```python
from build123d import *

# Parameters (mm, degrees)
BOSS_EXTRUDE1_DEPTH = 7.5
CIRPATTERN1_COUNT   = 20


with BuildPart() as part:
    # Sketch1 → Revolve1 (revolve)
    with BuildSketch(Plane(origin=(0, 0, 0), x_dir=(0, 0, -1), z_dir=(1, 0, 0)), mode=Mode.PRIVATE) as revolve1_sk:
        Polygon((-3.75, 7.5), (-3.75, 5.5), (3.75, 5.5), (3.75, 7.5), (4.25, 9), (5.4, 9), (5.4, 5.075), (5.8, 5.075), (5.8, 2.5), (-5.8, 2.5), (-5.8, 5.075), (-5.4, 5.075), (-5.4, 9), (-4.25, 9), align=None)
    revolve(revolve1_sk.sketch.rotate(Axis((0, 0, 0), (0, 0, -1)), 90), axis=Axis((0, 0, 0), (0, 0, -1)))

    # Sketch2 → Boss-Extrude1 (add)
    with BuildSketch(Plane.XY.offset(-3.75)):
        with BuildLine():
            ThreePointArc((0.499483204, 5.477272727), (0, 6), (-0.499483204, 5.477272727))
            ThreePointArc((-0.499483204, 5.477272727), (0, 5.5), (0.499483204, 5.477272727))
        make_face()
    boss_extrude1 = extrude(amount=BOSS_EXTRUDE1_DEPTH)

    # CirPattern1: Boss-Extrude1 ×20 about axis
    cirpattern1_axis = Axis((0, 0, 0), (0, 0, 1))
    for i in range(1, CIRPATTERN1_COUNT):
        add(boss_extrude1.rotate(cirpattern1_axis, i * 360 / CIRPATTERN1_COUNT))


solid = part.part
```
Geometry check sheet. Reference: the model listing, model coordinates, mm. A direction names the side the tool comes from. Coordinates: 2 decimals unless noted, no trailing zeros. Order: outer loops, then holes, each group sorted by start corner. A loop starts at its lowest first (then second) coordinate and runs counter-clockwise, first axis right, second up.
Item 1: Mould release check, pull along X, two halves, no side actions. Record for faces 4 (the cylindrical face through (-2.5, -0.1, 0.1)), 5 (the cylindrical face through (-6.633, -6.083, -4.833)), 6 (the flat face through (-4, 4, 5.4)): released by +X, released by -X, zero draft, split by the parting line, or undercut.
Item 2: Section check A-A (y = 0). Enter the section's corners in (x, z) (3 decimals), plus the area to 3 significant figures.
Item 3: Scan lines: line 1 along Z through (x, y) = (4.5, 4); line 2 along Y through (x, z) = (0, 1.25); line 3 along Y through (x, z) = (0.75, -2.25). Record each from-to range of solid material in increasing order.
Item 4: Tool access check on faces 1 (the flat face through (-4, -4, 3.75)), 2 (the flat face through (2, 2, -5.8)), 3 (the cylindrical face through (-4.027, 3.088, 5.597)). Record the directions out of +Z, -Z, +X, -X, +Y, -Y that give a thin tool (end or side, any length) a straight path to the whole face; none if there is none.
Item 5: Depth check by flat-ended pin: pin 1 (3 mm diameter, centred on x = 2, z = -4, fed in from -Y); pin 2 (1.5 mm diameter, centred on x = 1.5, z = -1, fed in from -Y); pin 3 (1 mm diameter, centred on y = -3.5, z = 1.5, fed in from +X); pin 4 (5 mm diameter, centred on x = -2.5, z = 4.5, fed in from +Y). Enter the tip coordinate at first touch or a pass-through.
Item 6: Section check B-B (z = -4.5). Enter the section's corners in (x, y).
Check sheet entries:
1. face 4: undercut
1. face 5: split by the parting line
1. face 6: zero draft
2. outline: (-9, -5.4) - (-5.075, -5.4) - (-5.075, -5.8) - (-2.5, -5.8) - (-2.5, 5.8) - (-5.075, 5.8) - (-5.075, 5.4) - (-9, 5.4) - (-9, 4.25) - (-7.5, 3.75) - (-6, 3.75) - (-6, -3.75) - (-7.5, -3.75) - (-9, -4.25) - close; (2.5, -5.8) - (5.075, -5.8) - (5.075, -5.4) - (9, -5.4) - (9, -4.25) - (7.5, -3.75) - (6, -3.75) - (6, 3.75) - (7.5, 3.75) - (9, 4.25) - (9, 5.4) - (5.075, 5.4) - (5.075, 5.8) - (2.5, 5.8) - close
2. area: 98.0 mm2
3. line 1: z = -5.4 to -3.75, 3.75 to 5.4
3. line 2: y = -6 to -2.5, 2.5 to 6
3. line 3: y = -5.45 to -2.38, 2.38 to 5.45
4. face 1: none
4. face 2: -Z, +X, -X, +Y, -Y
4. face 3: +Z
5. pin 1: stops at y = -8.98
5. pin 2: stops at y = -5.73
5. pin 3: stops at x = 4.95
5. pin 4: stops at y = 9
6. outline: circle Ø18 at (0, 0); hole circle Ø5 at (0, 0)
